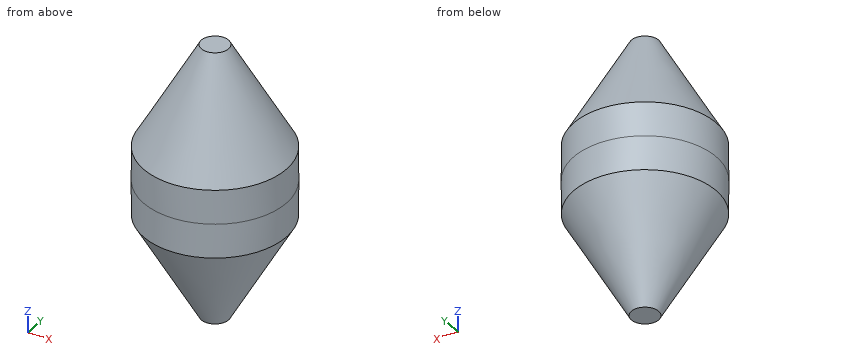
```python
from build123d import *

# Parameters (mm, degrees)
F0_R     = 13.335
F1_DEPTH = 6.35


with BuildPart() as f1:
    # F0 (on Top) → F1 (new body)
    with BuildSketch(Plane.XY):
        Circle(F0_R)
    extrude(amount=F1_DEPTH)

    # F4 (on Right) → F6 (revolve)
    with BuildSketch(Plane.YZ):
        Polygon((0, 25.4), (0, 6.35), (13.335, 6.35), (2.54, 25.4), align=None)
    revolve(axis=Axis((0, 0, 24.791185), (0, 0, 1)))

    # F7: F1 across plane


with BuildPart() as f1_1:
    add(f1.part)
    add(f1.part.mirror(Plane.XY))


solid = f1_1.part
```
Here's how the part is built. I have some questions about the finished solid (model axes, mm). Coordinates: 2 decimals unless noted, no trailing zeros. Write each loop counter-clockwise with the first axis right and the second up, starting at its lowest first coordinate (ties: lowest second). Pieces come first, ordered by that corner, then holes. Notation, with made-up numbers: (45.5, 31.25) -> (78.5, 31.25) arc R8 ccw to (78.5, 41.25) -> close; hole circle Ø10 at (75, 79.5). An arc over 180 degrees is marked (long way). Use a Markdown table: item, result. Add a question column.
(1) I'm going to push flat-ended pins straight in: P1, Ø6, axis at x = 9.5, z = 1, coming from the +Y side; P2, Ø2, axis at x = -6.5, y = -10.5, coming from the +Z side; P3, Ø4, axis at x = 4.5, z = -15, coming from the -Y side. Where does each tip first touch, or does it pass through?
(2) If we section it at A-A, the plane y = 0: Write out the boundary of the cut face in (x, z) (3 decimals), and give its area (3 significant figures).
(3) If we section it at C-C, the plane z = 11.5: Write out the boundary of the cut face in (x, y).
(4) Please list where these lines run through material, in increasing order: line 1 (Y direction, x = 0.5, z = -20.5); line 2 (Y direction, x = -7, z = -2); line 3 (X direction, y = -5.5, z = -5).
Outcome:
| question | item | result |
|---|---|---|
| 1 | P1 | stops at y = 11.64 |
| 1 | P2 | stops at z = 9.85 |
| 1 | P3 | stops at y = -8.74 |
| 2 | outline | (-13.335, -6.35) -> (-2.54, -25.4) -> (2.54, -25.4) -> (13.335, -6.35) -> (13.335, 6.35) -> (2.54, 25.4) -> (-2.54, 25.4) -> (-13.335, 6.35) -> close |
| 2 | area | 944 mm^2 |
| 3 | outline | circle Ø20.83 at (0, 0) |
| 4 | line 1 | y = -5.29 to 5.29 |
| 4 | line 2 | y = -11.35 to 11.35 |
| 4 | line 3 | x = -12.15 to 12.15 |
